For this review, take the finished solid that the model builds, in its own axes (mm). Coordinates: 2 decimals unless noted, no trailing zeros. Write each loop counter-clockwise with the first axis right and the second up, starting at its lowest first coordinate (ties: lowest second). Pieces come first, ordered by that corner, then holes.
1) We need section C-C on z = 1. Write out the cut boundary in (x, y).
2) We need section B-B on y = 0.8. Write out the cut boundary in (x, z).
3) We need section A-A on z = -7.15. Give the number of separate pieces and of enclosed holes in the cut face, then the cut area to 3 significant figures.
4) Insertion check: P1, Ø0.6, axis at y = 1, z = 9.5, coming from the -X side; P2, Ø1, axis at y = 0.5, z = 12.5, coming from the +X side; P3, Ø0.6, axis at x = -18.5, y = 1.5, coming from the -Z side. Each pin has a flat end and moves straight along its axis. Give the tip position at first contact, or say it passes through.
5) To check wall thickness, follow line 1 along X through (y, z) = (0.1, -25.15); line 2 along X through (y, z) = (1.75, 22.5); line 3 along Z through (x, y) = (16.5, 0.95). State the ranges of each line that lie inside material, in increasing order.
from build123d import *

# Parameters (mm, degrees)
SKETCH1_W            = 36
SKETCH1_H            = 62.2
BASE_SHAPE_DEPTH     = 2
CUTOUTS_REACH        = 37.989
SKETCH2_R            = 1.65
SKETCH2_W            = 0.5
SKETCH2_H            = 20.5
SKETCH3_W            = 1.5
SKETCH3_H            = 28.95
SKETCH3_H_2          = 12.75
EXTRA_SIZE_DEPTH     = 2
SKETCH4_R            = 3
SCREW_HEAD_CUT_DEPTH = 0.4
SCREW_CHAMFER_SIZE   = 1.35
FILLET1_R            = 4


with BuildPart() as part:
    # Sketch1 → Base shape (new body)
    with BuildSketch(Plane(origin=(0, 0, 0), x_dir=(1, 0, 0), z_dir=(0, 1, 0))):
        Rectangle(SKETCH1_W, SKETCH1_H)
    extrude(amount=BASE_SHAPE_DEPTH)

    # Sketch2 → Cutouts (cut, up to next)
    with BuildSketch(Plane(origin=(0, 2, 0), x_dir=(1, 0, 0), z_dir=(0, 1, 0)), mode=Mode.PRIVATE) as cutouts_sk1:
        with Locations(Location((-15.25, 7.15, 0), (0, 0, 270))):
            Circle(SKETCH2_R)
    cutouts_tool1 = extrude(cutouts_sk1.sketch, amount=-CUTOUTS_REACH, mode=Mode.PRIVATE) & part.part
    # Sketch2 → Cutouts (cut, up to next)
    with BuildSketch(Plane(origin=(0, 2, 0), x_dir=(1, 0, 0), z_dir=(0, 1, 0)), mode=Mode.PRIVATE) as cutouts_sk2:
        with Locations(Location((15.25, 7.15, 0), (0, 0, 270))):
            Circle(SKETCH2_R)
    cutouts_tool2 = extrude(cutouts_sk2.sketch, amount=-CUTOUTS_REACH, mode=Mode.PRIVATE) & part.part
    # Sketch2 → Cutouts (cut, up to next)
    with BuildSketch(Plane(origin=(0, 2, 0), x_dir=(1, 0, 0), z_dir=(0, 1, 0)), mode=Mode.PRIVATE) as cutouts_sk3:
        with Locations((17.75, -8.1)):
            Rectangle(SKETCH2_W, SKETCH2_H)
    cutouts_tool3 = extrude(cutouts_sk3.sketch, amount=-CUTOUTS_REACH, mode=Mode.PRIVATE) & part.part
    # Sketch2 → Cutouts (cut, up to next)
    with BuildSketch(Plane(origin=(0, 2, 0), x_dir=(1, 0, 0), z_dir=(0, 1, 0)), mode=Mode.PRIVATE) as cutouts_sk4:
        with Locations((-17.75, -8.1)):
            Rectangle(SKETCH2_W, SKETCH2_H)
    cutouts_tool4 = extrude(cutouts_sk4.sketch, amount=-CUTOUTS_REACH, mode=Mode.PRIVATE) & part.part
    # Sketch2 → Cutouts (cut, up to next)
    with BuildSketch(Plane(origin=(0, 2, 0), x_dir=(1, 0, 0), z_dir=(0, 1, 0)), mode=Mode.PRIVATE) as cutouts_sk5:
        with Locations(Location((-15.25, -23.35, 0), (0, 0, 270))):
            Circle(SKETCH2_R)
    cutouts_tool5 = extrude(cutouts_sk5.sketch, amount=-CUTOUTS_REACH, mode=Mode.PRIVATE) & part.part
    # Sketch2 → Cutouts (cut, up to next)
    with BuildSketch(Plane(origin=(0, 2, 0), x_dir=(1, 0, 0), z_dir=(0, 1, 0)), mode=Mode.PRIVATE) as cutouts_sk6:
        with Locations(Location((15.25, -23.35, 0), (0, 0, 270))):
            Circle(SKETCH2_R)
    cutouts_tool6 = extrude(cutouts_sk6.sketch, amount=-CUTOUTS_REACH, mode=Mode.PRIVATE) & part.part
    # Sketch2 → Cutouts (cut, up to next)
    with BuildSketch(Plane(origin=(0, 2, 0), x_dir=(1, 0, 0), z_dir=(0, 1, 0)), mode=Mode.PRIVATE) as cutouts_sk7:
        with Locations(Location((-15.25, 25.15, 0), (0, 0, 270))):
            Circle(SKETCH2_R)
    cutouts_tool7 = extrude(cutouts_sk7.sketch, amount=-CUTOUTS_REACH, mode=Mode.PRIVATE) & part.part
    # Sketch2 → Cutouts (cut, up to next)
    with BuildSketch(Plane(origin=(0, 2, 0), x_dir=(1, 0, 0), z_dir=(0, 1, 0)), mode=Mode.PRIVATE) as cutouts_sk8:
        with Locations(Location((15.25, 25.15, 0), (0, 0, 270))):
            Circle(SKETCH2_R)
    cutouts_tool8 = extrude(cutouts_sk8.sketch, amount=-CUTOUTS_REACH, mode=Mode.PRIVATE) & part.part
    add(cutouts_tool1.solids().sort_by_distance((-15.25, 2, -7.15))[0], mode=Mode.SUBTRACT)
    add(cutouts_tool2.solids().sort_by_distance((15.25, 2, -7.15))[0], mode=Mode.SUBTRACT)
    add(cutouts_tool3.solids().sort_by_distance((17.75, 2, 8.1))[0], mode=Mode.SUBTRACT)
    add(cutouts_tool4.solids().sort_by_distance((-17.75, 2, 8.1))[0], mode=Mode.SUBTRACT)
    add(cutouts_tool5.solids().sort_by_distance((-15.25, 2, 23.35))[0], mode=Mode.SUBTRACT)
    add(cutouts_tool6.solids().sort_by_distance((15.25, 2, 23.35))[0], mode=Mode.SUBTRACT)
    add(cutouts_tool7.solids().sort_by_distance((-15.25, 2, -25.15))[0], mode=Mode.SUBTRACT)
    add(cutouts_tool8.solids().sort_by_distance((15.25, 2, -25.15))[0], mode=Mode.SUBTRACT)

    # Sketch3 → Extra size (add)
    with BuildSketch(Plane.XZ):
        with Locations((-18.75, -16.625)):
            Rectangle(SKETCH3_W, SKETCH3_H)
        with Locations((18.75, -16.625)):
            Rectangle(SKETCH3_W, SKETCH3_H)
        with Locations((-18.75, 24.725)):
            Rectangle(SKETCH3_W, SKETCH3_H_2)
        with Locations((18.75, 24.725)):
            Rectangle(SKETCH3_W, SKETCH3_H_2)
        Polygon((19.5, 31.1), (19.5, 32.6), (-19.5, 32.6), (-19.5, 31.1), (-18, 31.1), (18, 31.1), align=None)
    extrude(amount=-EXTRA_SIZE_DEPTH)

    # Sketch4 → Screw head cut (cut)
    with BuildSketch(Plane(origin=(0, 0, 0), x_dir=(1, 0, 0), z_dir=(0, 1, 0))):
        with Locations(Location((-15.25, 25.15, 0), (0, 0, 270))):
            Circle(SKETCH4_R)
        with Locations(Location((15.25, 25.15, 0), (0, 0, 270))):
            Circle(SKETCH4_R)
        with Locations(Location((15.25, 7.15, 0), (0, 0, 270))):
            Circle(SKETCH4_R)
        with Locations(Location((-15.25, 7.15, 0), (0, 0, 270))):
            Circle(SKETCH4_R)
        with Locations(Location((-15.25, -23.35, 0), (0, 0, 270))):
            Circle(SKETCH4_R)
        with Locations(Location((15.25, -23.35, 0), (0, 0, 270))):
            Circle(SKETCH4_R)
    extrude(amount=SCREW_HEAD_CUT_DEPTH, mode=Mode.SUBTRACT)

    # Screw chamfer
    screw_chamfer_edges = [part.edges().sort_by_distance(p)[0] for p in [
        (-15.25, 0.4, -26.8),
        (15.25, 0.4, 21.7),
        (-15.25, 0.4, 21.7),
        (-15.25, 0.4, -8.8),
        (15.25, 0.4, -8.8),
        (15.25, 0.4, -26.8),
    ]]
    chamfer(screw_chamfer_edges, length=SCREW_CHAMFER_SIZE - 0.0001)  # a hair under: the kernel refuses the full size

    # Fillet1
    fillet1_edges = [part.edges().sort_by_distance(p)[0] for p in [
        (-19.5, 1, -31.1),
        (19.5, 1, -31.1),
    ]]
    fillet(fillet1_edges, radius=FILLET1_R)


solid = part.part
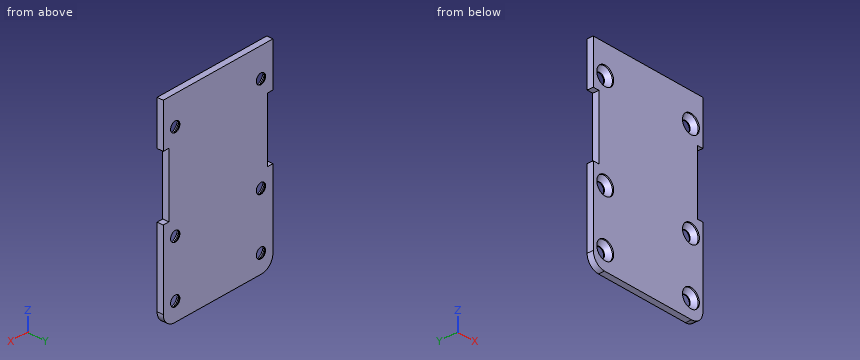
Result:
1. outline: (-17.5, 0) - (17.5, 0) - (17.5, 2) - (-17.5, 2) - close
2. outline: (-19.5, -27.1) arc R4 ccw to (-15.5, -31.1) - (15.5, -31.1) arc R4 ccw to (19.5, -27.1) - (19.5, -2.15) - (17.5, -2.15) - (17.5, 18.35) - (19.5, 18.35) - (19.5, 32.6) - (-19.5, 32.6) - (-19.5, 18.35) - (-17.5, 18.35) - (-17.5, -2.15) - (-19.5, -2.15) - close; hole circle Ø5.2 at (-15.25, -25.15); hole circle Ø5.2 at (-15.25, -7.15); hole circle Ø5.2 at (-15.25, 23.35); hole circle Ø5.2 at (15.25, -25.15); hole circle Ø5.2 at (15.25, -7.15); hole circle Ø5.2 at (15.25, 23.35)
3. separate pieces: 3
3. enclosed holes: 0
3. area: 59.0 mm2
4. P1: stops at x = -17.5
4. P2: stops at x = 17.5
4. P3: stops at z = -30.05
5. line 1: x = -19.5 to -18.25, -12.25 to 12.25, 18.25 to 19.5
5. line 2: x = -19.5 to -16.66, -13.84 to 13.84, 16.66 to 19.5
5. line 3: z = -30.97 to -27.26, -23.04 to -9.26, -5.04 to 21.24, 25.46 to 32.6
